Input: part model. Units: mm. Frame: model coordinates. Face numbers are marked on the shaded views. A direction names the side the tool comes from. Round coordinates to 2 decimals unless told otherwise and drop trailing zeros. Loops run counter-clockwise (first coordinate to the right, second up) from the corner with the lowest first, then second, coordinate; pieces in that order, holes last.
1) Section D-D, the plane y = 18.5. Return loops of the section in (x, z), and give its area (3 significant figures).
2) Section B-B, the plane z = 7. Return loops of the section in (x, y).
3) Ray query, line 1 along X through (y, z) = (4.5, -8.25); line 2 along Z through (x, y) = (41.5, 13.5); line 3 along X through (y, z) = (10.25, 4.5). Return the intervals inside material, ascending.
4) Section A-A, the plane y = 10. Return loops of the section in (x, z).
5) Section C-C, the plane x = 42. Return loops of the section in (y, z).
6) Access query for the marked faces 1, 2 and 3. Directions: +Z, -Z, +X, -X, +Y, -Y. A direction counts if a zero-diameter tool reaches every point of the face in a straight line with its end or side. Return the directions, or none.
7) First-contact query: pin 1 (1.5 mm diameter, centred on y = 15, z = -1.5, fed in from +X); pin 2 (6 mm diameter, centred on x = 34, z = 4, fed in from -Y); pin 3 (1.8 mm diameter, centred on x = 43.5, y = 9, fed in from -Z). Flat tips, straight axial feed; report the tip coordinate or a pass-through.
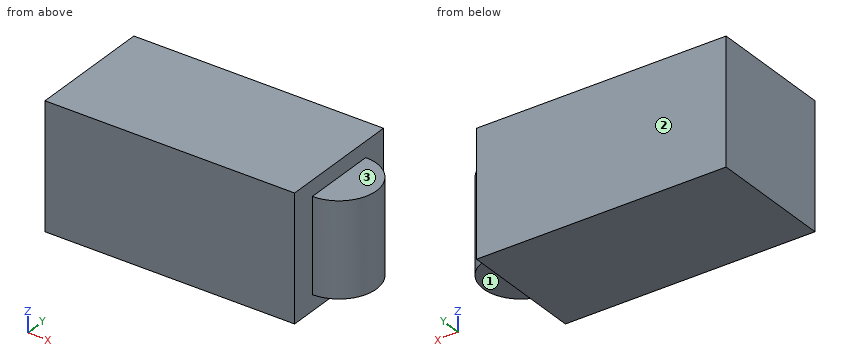
from build123d import *

# Parameters (mm, degrees)
SKETCH1_W           = 40
SKETCH1_H           = 20
BOSS_EXTRUDE1_DEPTH = 10
SKETCH2_R           = 6
BOSS_EXTRUDE2_DEPTH = 7.5


with BuildPart() as part:
    # Sketch1 → Boss-Extrude1 (new, symmetric)
    with BuildSketch(Plane.XY):
        with Locations((20, 10)):
            Rectangle(SKETCH1_W, SKETCH1_H)
    extrude(amount=BOSS_EXTRUDE1_DEPTH, both=True)

    # Sketch2 → Boss-Extrude2 (add, symmetric)
    with BuildSketch(Plane.XY):
        with Locations((40, 10)):
            Circle(SKETCH2_R)
    extrude(amount=BOSS_EXTRUDE2_DEPTH, both=True)


solid = part.part
Final values:
1. outline: (0, -10) - (40, -10) - (40, 10) - (0, 10) - close
1. area: 800 mm2
2. outline: (0, 0) - (40, 0) - (40, 4) arc R6 ccw to (40, 16) - (40, 20) - (0, 20) - close
3. line 1: x = 0 to 40
3. line 2: z = -7.5 to 7.5
3. line 3: x = 0 to 45.99
4. outline: (0, -10) - (40, -10) - (40, -7.5) - (46, -7.5) - (46, 7.5) - (40, 7.5) - (40, 10) - (0, 10) - close
5. outline: (4.34, -7.5) - (15.66, -7.5) - (15.66, 7.5) - (4.34, 7.5) - close
6. face 1: -Z, +X, +Y, -Y
6. face 2: +Z, -Z, +X, -X, +Y
6. face 3: +Z, +X, +Y, -Y
7. pin 1: stops at x = 44.24
7. pin 2: stops at y = 0
7. pin 3: stops at z = -7.5
